Part model, mm, in its own coordinate system. Face numbers are marked on the shaded views. A direction names the side the tool comes from. Give positions to 0.01 mm unless a question says otherwise; leave off trailing zeros. Write each loop counter-clockwise with the first axis right and the second up, starting at its lowest first coordinate (ties: lowest second). Pieces come first, ordered by that corner, then holes.
Autodesk Inventor part; units mm, degrees
ref_plane "YZ Plane" through (0, 0, 0) normal (1, 0, 0) x (0, 1, 0)
ref_plane "XZ Plane" through (0, 0, 0) normal (0, 1, 0) x (-1, 0, 0)
ref_plane "XY Plane" through (0, 0, 0) normal (0, 0, 1) x (1, 0, 0)
sketch "Sketch1" plane through (0, 0, 0) normal (0, 0, 1) x (1, 0, 0)
  line L0 (0, 0) -> (160.4518, 0)
  line L1 (160.4518, 0) -> (160.4518, 30.4038)
  line L2 (160.4518, 30.4038) -> (0, 30.4038)
  line L3 (0, 30.4038) -> (0, 0)
  line L4 (97.5982, 24.1046) -> (160.4518, 24.1046)
  line L5 (95.9612, 25.7556) -> (92.9894, 28.7528) construction
  line L6 (91.3524, 30.4038) -> (97.5982, 24.1046)
  dimension "d0" = 160.4518
  dimension "d1" = 30.4038
  dimension "d4" = 67.4624
  dimension "d5" = 1.651
  dimension "d8" = 64.4906
  dimension "d9" = 4.6482
  dimension "d10" = 6.2992
extrude "Extrusion1" add sketch "Sketch1" along normal blind 46.4312 contours L3 L2 L6 L4 L1 L0
fillet "Fillet1" radius 5.6642 2 edges at (91.3524, 30.4038, 23.2156) (97.5982, 24.1046, 23.2156)
chamfer "Chamfer1" distance 4.5974 distance2 4.0894 1 edges at (160.4518, 24.1046, 23.2156) measured on face at (140.2874, 24.1046, 15.4771)
chamfer "Chamfer3" distance 4.0894 distance2 6.4516 3 edges at (127.9065, 24.1046, 0) (94.4753, 27.2542, 0) (44.496, 30.4038, 0) measured on face at (86.4331, 8.0715, 0)
chamfer "Chamfer2" distance 4.0894 distance2 6.4516 3 edges at (127.9065, 24.1046, 46.4312) (94.4753, 27.2542, 46.4312) (44.496, 30.4038, 46.4312) measured on face at (86.4331, 8.0715, 46.4312)
chamfer "Chamfer4" distance 4.0894 distance2 4.5974 1 edges at (0, 30.4038, 23.2156) measured on face at (0, 10.1346, 28.8036)
chamfer "Chamfer5" distance 3.429 distance2 4.0132 1 edges at (0, 0, 23.2156) measured on face at (0, 17.5429, 30.9541)
chamfer "Chamfer6" distance 3.8862 distance2 6.3246 1 edges at (82.2325, 0, 46.4312) measured on face at (87.5035, 6.7349, 46.4312)
chamfer "Chamfer7" distance 4.0132 distance2 3.429 1 edges at (160.4518, 0, 20.0533) measured on face at (160.4518, 13.3435, 28.8459)
chamfer "Chamfer8" distance 3.8862 distance2 6.3246 1 edges at (80.518, 0, 0) measured on face at (86.3605, 6.7349, 0)
fillet "Fillet2" radius 3.175 12 edges at (0, 15.1003, 0) (2.2987, 28.3591, 3.2258) (0, 15.1003, 46.4312) (2.2987, 28.3591, 43.2054) (2.0066, 1.7145, 3.5343) (2.0066, 1.7145, 42.8969) (158.683, 1.9431, 3.1623) (160.4518, 12.0142, 0) (158.1531, 22.0599, 3.2258) (158.1531, 22.0599, 43.2054) (160.4518, 12.0142, 46.4312) (158.683, 1.9431, 43.2689)
sketch "Sketch2" plane through (0, 3.429, 43.2562) normal (-1, 0, 0) x (0, 0, 1)
  line L0 (-32.0153, 0.1) -> (-56.6979, 0.1) construction
  line L1 (-56.6979, 0.1) -> (-56.6979, 8.3256) construction
  line L2 (-56.6979, 8.3256) -> (-32.0153, 8.3256) construction
  line L3 (-32.0153, 8.3256) -> (-32.0153, 0.1) construction
  ellipse E0 centre (-40.1387, 8.5022) end of major axis (-39.8909, 8.2522) minor radius 0.0031 (-40.1387, 8.4978) -> (-39.8909, 8.2522) ccw construction
  line L4 (-48.8131, 12.2136) -> (-39.9668, 12.2136) construction
  line L5 (-39.9668, 12.2136) -> (-39.9668, 8.3256) construction
  line L6 (-39.9668, 8.3256) -> (-48.8131, 8.3256) construction
  line L7 (-48.8131, 8.3256) -> (-48.8131, 12.2136) construction
  line L8 (-38.1, 18.161) -> (-13.4174, 18.161)
  line L9 (-13.4174, 18.161) -> (-13.4174, 9.9354)
  line L10 (-13.4174, 9.9354) -> (-38.1, 9.9354)
  line L11 (-38.1, 9.9354) -> (-38.1, 18.161)
  line L12 (-30.2152, 9.9354) -> (-21.3689, 9.9354)
  line L13 (-21.3689, 9.9354) -> (-21.3689, 6.0474)
  line L14 (-21.3689, 6.0474) -> (-30.2152, 6.0474)
  line L15 (-30.2152, 6.0474) -> (-30.2152, 9.9354)
  line L16 (-5.4645, 26.9748) -> (-34.6167, 26.9748)
  line L17 (-43.2562, 22.8854) -> (-43.2562, 0.4572)
  point P0 (-43.2562, -3.429)
  point P1 (-21.3689, 9.9354)
  dimension "d40" = 8.8464
  dimension "d41" = 8.2256
  dimension "d42" = 24.6826
  dimension "d43" = 3.888
  dimension "d44" = 7.8848
  dimension "d45" = 8.2256
  dimension "d46" = 24.6826
  dimension "d47" = 7.8848
  dimension "d48" = 3.888
  dimension "d49" = 8.8464
  dimension "d50" = 7.9515
  dimension "d51" = 7.9515
  dimension "d52" = 8.8138
  dimension "d53" = 5.1562
extrude "Extrusion2" add sketch "Sketch2" along normal blind 15.875
equation "\"d45\" = d41"
equation "\"d46\" = d42"
equation "\"d47\" = d44"
equation "\"d48\" = d43"
equation "\"d49\" = d40"
properties part number "V5 Simple Battery"
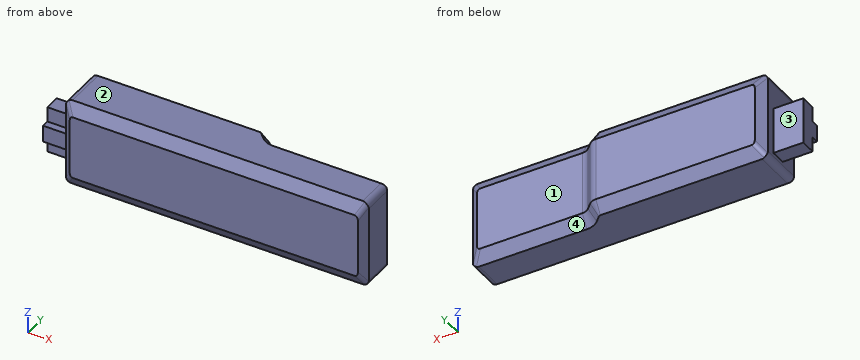
1) Saw through at C-C, the plane z = 15.5. Write the cut outline in (x, y) (3 decimals), then the cut area to 3 significant figures.
Answers follow:
outline: (-15.875, 9.476) - (0, 9.476) - (0, 3.429) - (4.013, 0) - (157.023, 0) - (160.452, 4.013) - (160.452, 20.015) - (155.854, 24.105) - (99.959, 24.105) arc R5.664 cw to (95.936, 25.781) - (93.014, 28.728) arc R5.664 ccw to (88.992, 30.404) - (4.597, 30.404) - (0, 26.314) - (0, 21.59) - (-15.875, 21.59) - close
area: 4,620 mm2
2) Pin check, flat tips, straight feed: pin 1 Ø4.5 at (x, y) = (-9, 10.5) entering from -Z; pin 2 Ø6.5 at (x, y) = (-9.5, 18.5) entering from -Z; pin 3 Ø3 at (x, y) = (-5.5, 12.5) entering from +Z. Stop position of each tip, or through.
Answers follow:
pin 1: stops at z = 13.04
pin 2: stops at z = 5.16
pin 3: stops at z = 29.84
3) Saw through at D-D, the plane y = 18.5. Write the cut outline in (x, z) (3 decimals).
Answers follow:
outline: (-15.875, 5.156) - (0, 5.156) - (0, 3.175) arc R3.175 ccw to (3.175, 0) - (157.277, 0) arc R3.175 ccw to (160.452, 3.175) - (160.452, 43.256) arc R3.175 ccw to (157.277, 46.431) - (3.175, 46.431) arc R3.175 ccw to (0, 43.256) - (0, 29.839) - (-15.875, 29.839) - close
4) Wall check: L1, parallel to X at y = 10, z = 12.5; L2, parallel to Y at x = 93, z = 21; L3, parallel to Y at x = 107.5, z = 36.5. Give the ranges that are in metal, low to high.
Answers follow:
L1: x = 0 to 160.45
L2: y = 0 to 28.74
L3: y = 0 to 24.1
5) Saw through at A-A, the plane x = 142. Write the cut outline in (y, z).
Answers follow:
outline: (0, 6.32) - (3.89, 0) - (20.02, 0) - (24.1, 6.45) - (24.1, 39.98) - (20.02, 46.43) - (3.89, 46.43) - (0, 40.11) - close
6) Saw through at B-B, the plane y = 6. Write the cut outline in (x, z) (3 decimals), then the cut area to 3 significant figures.
Answers follow:
outline: (0, 3.175) arc R3.175 ccw to (3.175, 0) - (157.277, 0) arc R3.175 ccw to (160.452, 3.175) - (160.452, 43.256) arc R3.175 ccw to (157.277, 46.431) - (3.175, 46.431) arc R3.175 ccw to (0, 43.256) - close
area: 7,440 mm2
7) 3-axis set-ups, long thin cutter, end or side, ignore diameter. For the marked faces 1, 2, 3 and 4: which of +Z, -Z, +X, -X, +Y, -Y reach the whole face in a straight line?
Answers follow:
face 1: +Z, -Z, +X, +Y
face 2: +Z, +X, -X, +Y, -Y
face 3: +Z, -Z, -X, +Y
face 4: -Z, +X, +Y
